```python
from build123d import *

# Parameters (mm, degrees)
F1_DEPTH = 71.12
F2_DEPTH = 52.324
F3_SIZE  = 5.08
F4_R     = 8.142383265


with BuildPart() as f1:
    # F0 (on Top) → F1 (new body)
    with BuildSketch(Plane.XY):
        Polygon((7.5089540333, 17.2860901803), (-12.2935976833, 22.5921664387), (2.4708837736, -16.8182179332), (39.9978423606, 4.8479831407), align=None)
    extrude(amount=F1_DEPTH)

    # F2 (add): a face of the model
    f2_faces = [f1.faces().sort_by_distance(p)[0] for p in [
        (21.2343630671, -5.9851173963, 35.56),
    ]]
    extrude(f2_faces, amount=F2_DEPTH)

    # F3
    f3_edges = [f1.edges().sort_by_distance(p)[0] for p in [
        (39.997842, 4.847983, 35.56),
    ]]
    chamfer(f3_edges, length=F3_SIZE)

    # F4
    f4_edges = [f1.edges().sort_by_distance(p)[0] for p in [
        (-12.293598, 22.592166, 35.56),
    ]]
    fillet(f4_edges, radius=F4_R)


solid = f1.part
```
Check sheet for the modelled part. Datum: model origin and axes. Units: mm. Round coordinates to 2 decimals unless told otherwise and drop trailing zeros. Loops run counter-clockwise (first coordinate to the right, second up) from the corner with the lowest first, then second, coordinate; pieces in that order, holes last. Notation, with made-up numbers: (-13.75, 80.5) - (0.25, 80.5) arc R36 cw to (0.25, 116.5) - close; hole circle Ø9 at (-18.75, -38). An arc over 180 degrees is marked (long way). Answer as a JSON object with one key per item and string values. Group by question number.
Q1. Sectioned sample at C-C, the plane y = 5.5. Enter the section's corners in (x, z).
Q2. Sectioned sample at B-B, the plane x = 18.5. Enter the section's corners in (y, z).
Q3. Gauge pin test, flat ends, axial feed: P1, Ø5, axis at y = 4.5, z = 57.5, coming from the -X side; P2, Ø1.5, axis at y = -43, z = 18, coming from the -X side; P3, Ø1.5, axis at x = 22, z = 61.5, coming from the +Y side. Record the tip position at first contact, or that the pin passes through.
Q4. Sectioned sample at A-A, the plane z = 34. Enter the section's corners in (x, y), plus the area to 3 significant figures.
Q5. Scan lines: line 1 along Y through (x, z) = (28, 15.5); line 2 along X through (y, z) = (-47, 45.5); line 3 along Y through (x, z) = (4.5, 30). Record each from-to range of solid material in increasing order. Write a range as [from, to].
Solution:
{
 "1": {"outline": "(-5.89, 0) - (36.62, 0) - (36.62, 71.12) - (-5.89, 71.12) - close"},
 "2": {"outline": "(-44.58, 0) - (13.08, 0) - (13.08, 71.12) - (-44.58, 71.12) - close"},
 "3": {"P1": "stops at x = -6.45", "P2": "stops at x = 17.15", "P3": "stops at y = 12.03"},
 "4": {"outline": "(-6.74, 7.78) - (2.47, -16.82) - (28.63, -62.13) - (66.16, -40.47) - (42.54, 0.45) - (35.25, 6.66) - (7.51, 17.29) - (2.99, 18.5) arc R8.14 ccw to start", "area": "3,140 mm²"},
 "5": {"line 1": "y = [-61.04, 9.44]", "line 2": "x = [19.9, 54.84]", "line 3": "y = [-20.33, 18.09]"}
}
